Input: part model. Units: mm. Frame: model coordinates. A direction names the side the tool comes from. Coordinates: 2 decimals unless noted, no trailing zeros. Order: outer loops, then holes, each group sorted by start corner. A loop starts at its lowest first (then second) coordinate and runs counter-clockwise, first axis right, second up. Notation, with made-up numbers: M 10.25,65 L 33.25,65 A19 ccw 33.25,95 Z; hole C 14.25,40.5 d8. An arc over 180 degrees is marked long. One line per item, written item: value.
```python
from build123d import *

# Parameters (mm, degrees)
SKETCH1_W                      = 45
SKETCH1_H                      = 22
BASE_FLANGE1_DEPTH             = 2
EDGE_FLANGE1_STRIP_W           = 10
EDGE_FLANGE1_STRIP_H           = 2
EDGE_FLANGE1_STRIP_CUT_DEPTH   = 22
EDGE_FLANGE1_STRIP_2_W         = 10
EDGE_FLANGE1_STRIP_2_H         = 2
EDGE_FLANGE1_STRIP_CUT_2_DEPTH = 22
EDGE_FLANGE1_DEPTH             = 22
EDGE_FLANGE1_PROFILE_W         = 110
EDGE_FLANGE1_PROFILE_H         = 17
EDGE_FLANGE1_FLAT_DEPTH        = 2
EDGE_FLANGE1_BEND_DEPTH        = 22
EDGE_FLANGE1_PROFILE_2_W       = 110
EDGE_FLANGE1_PROFILE_2_H       = 17
EDGE_FLANGE1_FLAT_2_DEPTH      = 2
SKETCH24_R                     = 3.75
CUT_EXTRUDE1_DEPTH             = 10
CUT_EXTRUDE2_START             = -10
SKETCH25_R                     = 3.75
CUT_EXTRUDE2_DEPTH             = 10
SKETCH28_R                     = 1.75
CUT_EXTRUDE3_DEPTH             = 121.203993278
SKETCH29_W                     = 23
SKETCH29_H                     = 12
CUT_EXTRUDE4_DEPTH             = 10
CHAMFER1_SIZE                  = 2
CHAMFER2_SIZE                  = 10


# Sheet-metal steps are written as plain solids
with BuildPart() as part:
    # Sketch1 → Base-Flange1 (new body)
    with BuildSketch(Plane(origin=(0, 0, 0), x_dir=(1, 0, 0), z_dir=(0, 1, 0))):
        with Locations((22.5, 11)):
            Rectangle(SKETCH1_W, SKETCH1_H)
    extrude(amount=BASE_FLANGE1_DEPTH)

    # Edge-Flange1 strip (across the edge) → Edge-Flange1 strip cut (cut)
    with BuildSketch(Plane(origin=(45, 0, -22), x_dir=(-1, 0, 0), z_dir=(0, 0, 1))):
        with Locations((-2, -1)):
            Rectangle(EDGE_FLANGE1_STRIP_W, EDGE_FLANGE1_STRIP_H)
    extrude(amount=EDGE_FLANGE1_STRIP_CUT_DEPTH, mode=Mode.SUBTRACT)

    # Edge-Flange1 strip 2 (across the edge) → Edge-Flange1 strip cut 2 (cut)
    with BuildSketch(Plane(origin=(0, 0, 0), x_dir=(1, 0, 0), z_dir=(0, 0, -1))):
        with Locations((-2, -1)):
            Rectangle(EDGE_FLANGE1_STRIP_2_W, EDGE_FLANGE1_STRIP_2_H)
    extrude(amount=EDGE_FLANGE1_STRIP_CUT_2_DEPTH, mode=Mode.SUBTRACT)

    # Edge-Flange1 bend section (across the edge) → Edge-Flange1 (add)
    with BuildSketch(Plane(origin=(45, 0, -22), x_dir=(-1, 0, 0), z_dir=(0, 0, 1))):
        with BuildLine():
            Line((0, 1), (2, 1))
            ThreePointArc((2, 1), (2.292893219, 0.292893219), (3, 0))
            Line((3, 0), (3, -2))
            ThreePointArc((3, -2), (0.878679656, -1.121320344), (0, 1))
        make_face()
    extrude(amount=EDGE_FLANGE1_DEPTH)

    # Edge-Flange1 profile (on flange) → Edge-Flange1 flat (add)
    with BuildSketch(Plane(origin=(45, 0, 0), x_dir=(0, 0, 1), z_dir=(1, 0, 0))):
        with Locations((-55, 9.5)):
            Rectangle(EDGE_FLANGE1_PROFILE_W, EDGE_FLANGE1_PROFILE_H)
    extrude(amount=-EDGE_FLANGE1_FLAT_DEPTH)

    # Edge-Flange1 bend section 2 (across the edge) → Edge-Flange1 bend (add)
    with BuildSketch(Plane(origin=(0, 0, 0), x_dir=(1, 0, 0), z_dir=(0, 0, -1))):
        with BuildLine():
            Line((0, 1), (2, 1))
            ThreePointArc((2, 1), (2.292893219, 0.292893219), (3, 0))
            Line((3, 0), (3, -2))
            ThreePointArc((3, -2), (0.878679656, -1.121320344), (0, 1))
        make_face()
    extrude(amount=EDGE_FLANGE1_BEND_DEPTH)

    # Edge-Flange1 profile 2 (on flange) → Edge-Flange1 flat 2 (add)
    with BuildSketch(Plane(origin=(0, 0, 0), x_dir=(0, 0, -1), z_dir=(-1, 0, 0))):
        with Locations((55, 9.5)):
            Rectangle(EDGE_FLANGE1_PROFILE_2_W, EDGE_FLANGE1_PROFILE_2_H)
    extrude(amount=-EDGE_FLANGE1_FLAT_2_DEPTH)

    # Sketch24 → Cut-Extrude1 (cut)
    with BuildSketch(Plane(origin=(45, 0, 0), x_dir=(0, 0, -1), z_dir=(1, 0, 0))):
        with Locations(Location((90, -9.5, 0), (0, 0, 90))):
            Circle(SKETCH24_R)
    extrude(amount=-CUT_EXTRUDE1_DEPTH, mode=Mode.SUBTRACT)

    # Sketch25 → Cut-Extrude2 (cut)
    with BuildSketch(Plane.ZY.offset(CUT_EXTRUDE2_START)):
        with Locations(Location((-90, -9.5, 0), (0, 0, 90))):
            Circle(SKETCH25_R)
    extrude(amount=CUT_EXTRUDE2_DEPTH, mode=Mode.SUBTRACT)

    # Sketch28 → Cut-Extrude3 (cut, through all)
    with BuildSketch(Plane.ZY):
        with Locations(Location((-55, -9.5, 0), (0, 0, 270))):
            Circle(SKETCH28_R)
    extrude(amount=-CUT_EXTRUDE3_DEPTH, mode=Mode.SUBTRACT)

    # Sketch29 → Cut-Extrude4 (cut)
    with BuildSketch(Plane(origin=(0, 2, 0), x_dir=(1, 0, 0), z_dir=(0, 1, 0))):
        with Locations((22.5, 11)):
            Rectangle(SKETCH29_W, SKETCH29_H)
    extrude(amount=-CUT_EXTRUDE4_DEPTH, mode=Mode.SUBTRACT)

    # Chamfer1
    chamfer1_edges = [part.edges().sort_by_distance(p)[0] for p in [
        (44, -1, -110),
        (44, -18, -110),
        (1, -1, -110),
        (1, -18, -110),
    ]]
    chamfer(chamfer1_edges, length=CHAMFER1_SIZE)

    # Chamfer2
    chamfer2_edges = [part.edges().sort_by_distance(p)[0] for p in [
        (44, -18, 0),
        (1, -18, 0),
    ]]
    chamfer(chamfer2_edges, length=CHAMFER2_SIZE)


solid = part.part
```
(1) First-contact query: pin 1 (8 mm diameter, centred on x = 27.5, y = -0.5, fed in from +Z); pin 2 (1.5 mm diameter, centred on x = 33.5, y = 1, fed in from -Z); pin 3 (6.5 mm diameter, centred on x = 27, z = -11, fed in from -Y); pin 4 (0.6 mm diameter, centred on y = 1, z = -8.5, fed in from +X). Flat tips, straight axial feed; report the tip coordinate or a pass-through.
Data:
pin 1: stops at z = 0
pin 2: stops at z = -22
pin 3: passes through
pin 4: stops at x = 44.47
(2) Access query for faces 1 (the flat face through (22, 0, -4)), 2 (the flat face through (34, 1, -11)), 3 (the flat face through (1, -1, -64)). Directions: +Z, -Z, +X, -X, +Y, -Y. A direction counts if a zero-diameter tool reaches every point of the face in a straight line with its end or side. Return the directions, or none.
Data:
face 1: +Z, -Z, -Y
face 2: +Y, -Y
face 3: -Z, +X, -X, +Y
(3) Ray query, line 1 (X direction, y = -16.25, z = -90); line 2 (Z direction, x = 1.25, y = -9.5); line 3 (Z direction, x = 17, y = 1.25). Return the intervals inside material, ascending. Write a range as from..to.
Data:
line 1: x = 0..2, 43..45
line 2: z = -110..-93.75, -86.25..-56.75, -53.25..-1.5
line 3: z = -22..-17, -5..0
(4) Cut plane D-D on z = -34. Output: boundary loops of the cut face in (x, y).
Data:
outline: M 0,-18 L 2,-18 L 2,-1 L 0,-1 Z; M 43,-18 L 45,-18 L 45,-1 L 43,-1 Z
(5) Draft query along Y for faces 4 (the flat face through (22, 1, -17)), 5 (the flat face through (44, -1, -66)), 6 (the cylindrical face through (1.014, -9.988, -93.718)), 7 (the cylindrical face through (0.99, -9.12, -56.71)). Return one class per face: released by +Y, released by -Y, zero draft, split by the parting line, or undercut.
Data:
face 4: zero draft
face 5: released by +Y
face 6: undercut
face 7: undercut
(6) Cut plane B-B on z = -90. Output: boundary loops of the cut face in (x, y).
Data:
outline: M 0,-18 L 2,-18 L 2,-13.25 L 0,-13.25 Z; M 0,-5.75 L 2,-5.75 L 2,-1 L 0,-1 Z; M 43,-18 L 45,-18 L 45,-13.25 L 43,-13.25 Z; M 43,-5.75 L 45,-5.75 L 45,-1 L 43,-1 Z
(7) Cut plane C-C on y = -9.5. Output: boundary loops of the cut face in (x, z), plus the area to 3 significant figures.
Data:
outline: M 0,-110 L 2,-110 L 2,-93.75 L 0,-93.75 Z; M 0,-86.25 L 2,-86.25 L 2,-56.75 L 0,-56.75 Z; M 0,-53.25 L 2,-53.25 L 2,-1.5 L 0,-1.5 Z; M 43,-110 L 45,-110 L 45,-93.75 L 43,-93.75 Z; M 43,-86.25 L 45,-86.25 L 45,-56.75 L 43,-56.75 Z; M 43,-53.25 L 45,-53.25 L 45,-1.5 L 43,-1.5 Z
area: 390 mm2
(8) Cut plane A-A on x = 20.5. Output: boundary loops of the cut face in (y, z), plus the area to 3 significant figures.
Data:
outline: M 0,-22 L 2,-22 L 2,-17 L 0,-17 Z; M 0,-5 L 2,-5 L 2,0 L 0,0 Z
area: 20.0 mm2
